from build123d import *

# Parameters (mm, degrees)
SKETCH1_R           = 1.27
BOSS_EXTRUDE1_DEPTH = 0.889


with BuildPart() as part:
    # Sketch1 → Boss-Extrude1 (new body)
    with BuildSketch(Plane.XY):
        with BuildLine():
            Line((-4.547993368, 7.962766742), (-3.531993368, 0.850766742))
            ThreePointArc((-3.531993368, 0.850766742), (-2.264773091, 0.726570958), (-1.1995543, 0.029017555))
            ThreePointArc((-1.1995543, 0.029017555), (1.223134016, 1.819786094), (-0.798867095, 4.053120405))
            ThreePointArc((-0.798867095, 4.053120405), (-2.550299683, 5.854814329), (-2.477808037, 8.36645962))
            ThreePointArc((-2.477808037, 8.36645962), (-0.021575309, 9.082238313), (1.232714018, 6.852400507))
            ThreePointArc((1.232714018, 6.852400507), (2.205993955, 5.627515221), (3.765914813, 5.508080224))
            Line((3.765914813, 5.508080224), (3.562714813, -9.122319776))
            ThreePointArc((3.562714813, -9.122319776), (4.52052525, -9.888145198), (5.331956505, -8.968651464))
            Line((5.331956505, -8.968651464), (4.747756505, 6.372948536))
            Line((4.747756505, 6.372948536), (2.846185733, 6.372948536))
            Line((2.846185733, 6.372948536), (2.490585733, 8.963748536))
            ThreePointArc((2.490585733, 8.963748536), (-1.349608466, 10.719754973), (-4.547993368, 7.962766742))
        make_face()
        with Locations((-0.814199649, 2.021120405)):
            Circle(SKETCH1_R, mode=Mode.SUBTRACT)
    extrude(amount=BOSS_EXTRUDE1_DEPTH)


solid = part.part
Input: part model. Units: mm. Frame: model coordinates. A direction names the side the tool comes from. Round coordinates to 2 decimals unless told otherwise and drop trailing zeros. Order: outer loops, then holes, each group sorted by start corner. A loop starts at its lowest first (then second) coordinate and runs counter-clockwise, first axis right, second up. Notation, with made-up numbers: (32.25, -27.5) - (84.25, -27.5) arc R15 ccw to (84.25, -9.5) - close; hole circle Ø5 at (-20, 43.25). An arc over 180 degrees is marked (long way). Answer as a JSON object with one key per item and string values. Group by question number.
(1) Cut plane D-D (z = 0.35). Return loops of the section in (x, y).
(2) Reachability of faces 1 (the face through (-2.537, 5.821, 0.438)), 2 (the face through (0.7, 2.8, 0.889)), 3 (the face through (3.8, 6.373, 0.4)) from +Z, -Z, +X, -X, +Y, -Y: full face, straight path, thin tool, end or side. Return the list, or none.
(3) Draft query along Y for faces 4 (the face through (0.7, 2.8, 0)), 5 (the face through (1.218, 1.773, 0.438)), 6 (the face through (5.044, -1.405, 0.438)). Return one class per face: released by +Y, released by -Y, zero draft, split by the parting line, or undercut.
(4) Pin query (flat end, axial travel): P1, Ø5, axis at x = -0.5, y = -3, coming from the +Z side. Return the tip coordinate at first contact, or that it passes through.
(5) Cut plane B-B (x = -1). Return loops of the section in (y, z).
(6) Cut plane A-A (x = 0.75). Return loops of the section in (y, z), then the cut area to 3 significant figures.
(7) Cut plane C-C (y = 4.5). Return loops of the section in (x, z).
(8) Material intervals for probe 1 along X at (y, z) = (2, 0.45); probe 2 along X at (y, z) = (1.75, 0.5); probe 3 along Y at (x, z) = (-1, 0.4), sorted ascending. Write a range as from..to.
Here are the results:
{
 "1": {"outline": "(-4.55, 7.96) - (-3.53, 0.85) arc R2.67 cw to (-1.2, 0.03) arc R2.03 ccw (long way) to (-0.8, 4.05) arc R3.23 cw to (-2.48, 8.37) arc R2.06 cw to (1.23, 6.85) arc R1.96 ccw to (3.77, 5.51) - (3.56, -9.12) arc R0.89 ccw to (5.33, -8.97) - (4.75, 6.37) - (2.85, 6.37) - (2.49, 8.96) arc R3.91 ccw to start; hole circle Ø2.54 at (-0.81, 2.02)"},
 "2": {"face 1": "+Z, -Z", "face 2": "+Z, +X, -X, +Y, -Y", "face 3": "+Z, -Z, +X, +Y"},
 "3": {"face 4": "zero draft", "face 5": "undercut", "face 6": "released by +Y"},
 "4": {"P1": "passes through"},
 "5": {"outline": "(0, 0) - (0.76, 0) - (0.76, 0.89) - (0, 0.89) - close; (3.28, 0) - (4.15, 0) - (4.15, 0.89) - (3.28, 0.89) - close; (9.22, 0) - (10.75, 0) - (10.75, 0.89) - (9.22, 0.89) - close"},
 "6": {"outline": "(0.71, 0) - (3.34, 0) - (3.34, 0.89) - (0.71, 0.89) - close; (8.53, 0) - (10.44, 0) - (10.44, 0.89) - (8.53, 0.89) - close", "area": "4.03 mm^2"},
 "7": {"outline": "(-4.05, 0) - (-1.55, 0) - (-1.55, 0.89) - (-4.05, 0.89) - close; (3.75, 0) - (4.82, 0) - (4.82, 0.89) - (3.75, 0.89) - close"},
 "8": {"probe 1": "x = -3.7..-2.08, 0.46..1.23, 3.72..4.91", "probe 2": "x = -3.66..-2.05, 0.43..1.21, 3.71..4.92", "probe 3": "y = 0..0.76, 3.28..4.15, 9.22..10.75"}
}
